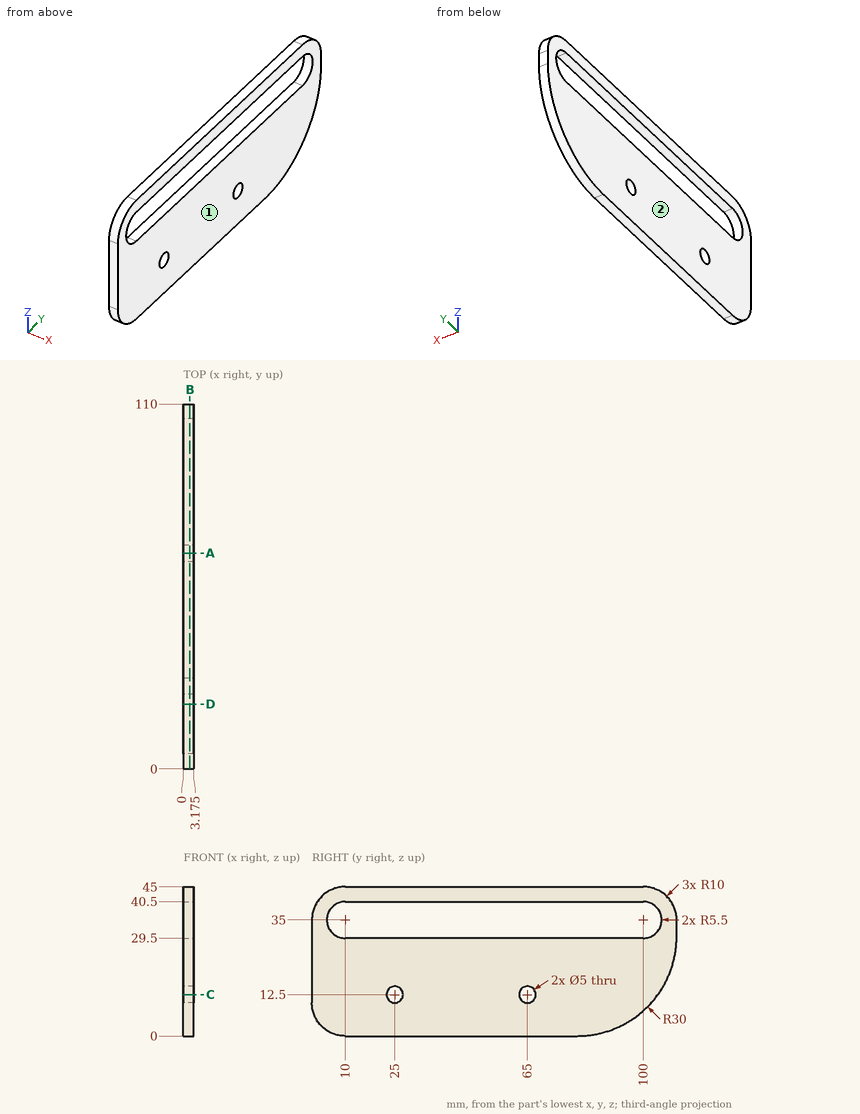
Answer from the drawing. Dimensions are ordinates in mm from the lowest x, y and z of the part. Give positions to 0.01 mm unless a question says otherwise; leave off trailing zeros. Order: outer loops, then holes, each group sorted by start corner. A loop starts at its lowest first (then second) coordinate and runs counter-clockwise, first axis right, second up.
Item 1: The part is cut by section A-A, the plane y = 65. Give the vertices of the cut face in (x, z) (3 decimals).
From the geometry:
outline: (0, 0) - (3.175, 0) - (3.175, 10) - (0, 10) - close; (0, 15) - (3.175, 15) - (3.175, 29.5) - (0, 29.5) - close; (0, 40.5) - (3.175, 40.5) - (3.175, 45) - (0, 45) - close
Item 2: The part is cut by section D-D, the plane y = 19.5. Give the vertices of the cut face in (x, z) (3 decimals), and give its area (3 significant figures).
From the geometry:
outline: (0, 0) - (3.175, 0) - (3.175, 29.5) - (0, 29.5) - close; (0, 40.5) - (3.175, 40.5) - (3.175, 45) - (0, 45) - close
area: 108 mm2
Item 3: The part is cut by section C-C, the plane z = 12.5. Give the vertices of the cut face in (x, y) (3 decimals), and give its area (3 significant figures).
From the geometry:
outline: (0, 0) - (3.175, 0) - (3.175, 22.5) - (0, 22.5) - close; (0, 27.5) - (3.175, 27.5) - (3.175, 62.5) - (0, 62.5) - close; (0, 67.5) - (3.175, 67.5) - (3.175, 104.367) - (0, 104.367) - close
area: 300 mm2
Item 4: For a pull along X with two mould halves and no side action, classify the marked faces 1 and 2 as pulls with the +X half, pulls with the -X half, needs draft (parallel to the pull), parting line crosses it, or undercut.
From the geometry:
face 1: pulls with the +X half
face 2: pulls with the -X half
Item 5: Find the intervals of material crossed by probe 1 along Z at (x, y) = (2.5, 65); probe 2 along Z at (x, y) = (2.85, 68); probe 3 along Z at (x, y) = (1.3, 63), in increasing order.
From the geometry:
probe 1: z = 0 to 10, 15 to 29.5, 40.5 to 45
probe 2: z = 0 to 29.5, 40.5 to 45
probe 3: z = 0 to 11, 14 to 29.5, 40.5 to 45
Item 6: The part is cut by section B-B, the plane x = 1.95. Give the vertices of the cut face in (y, z), and give its area (3 significant figures).
From the geometry:
outline: (0, 10) arc R10 ccw to (10, 0) - (80, 0) arc R30 ccw to (110, 30) - (110, 35) arc R10 ccw to (100, 45) - (10, 45) arc R10 ccw to (0, 35) - close; hole (10, 29.5) - (100, 29.5) arc R5.5 ccw to (100, 40.5) - (10, 40.5) arc R5.5 ccw to start; hole circle Ø5 at (25, 12.5); hole circle Ø5 at (65, 12.5)
area: 3,570 mm2
